from build123d import *

# Parameters (mm, degrees)
SKETCH1_R               = 6.35
BOSS_EXTRUDE1_DEPTH     = 25.4
CUT_EXTRUDE2_DEPTH      = 27.940768363
CUT_EXTRUDE2_DEPTH_BACK = 12.7
SKETCH3_R               = 4
SKETCH6_R               = 4.0005
CUT_EXTRUDE5_DEPTH      = 12.7
SKETCH4_R               = 1.1303
CUT_EXTRUDE3_DEPTH      = 6.35
SKETCH7_R               = 3.175
CUT_EXTRUDE6_DEPTH      = 12.7


with BuildPart() as part:
    # Sketch1 → Boss-Extrude1 (new body)
    with BuildSketch(Plane(origin=(0, 0, 0), x_dir=(1, 0, 0), z_dir=(0, 1, 0))):
        with Locations(Location((0, 0, 0), (0, 0, 270))):
            Circle(SKETCH1_R)
    extrude(amount=BOSS_EXTRUDE1_DEPTH)

    # Sketch3 → Cut-Extrude2 (cut, two sides: drawn at the far end of the back side and taken through both)
    with BuildSketch(Plane.XZ.offset(-CUT_EXTRUDE2_DEPTH_BACK)):
        with Locations(Location((0, 0, 0), (0, 0, 90))):
            Circle(SKETCH3_R)
    extrude(amount=CUT_EXTRUDE2_DEPTH + CUT_EXTRUDE2_DEPTH_BACK, mode=Mode.SUBTRACT)

    # Sketch6 → Cut-Extrude5 (cut)
    with BuildSketch(Plane(origin=(0, 0, 0), x_dir=(-1, 0, 0), z_dir=(0, -1, 0))):
        with Locations(Location((0, 0, 0), (0, 0, 90))):
            Circle(SKETCH6_R)
    extrude(amount=-CUT_EXTRUDE5_DEPTH, mode=Mode.SUBTRACT)

    # Sketch4 → Cut-Extrude3 (cut)
    with BuildSketch(Plane.XY.offset(6.35)):
        with Locations((0, 6.35)):
            Circle(SKETCH4_R)
        with Locations((0, 19.05)):
            Circle(SKETCH4_R)
    extrude(amount=-CUT_EXTRUDE3_DEPTH, mode=Mode.SUBTRACT)

    # Sketch7 → Cut-Extrude6 (cut)
    with BuildSketch(Plane(origin=(0, 25.4, 0), x_dir=(1, 0, 0), z_dir=(0, 1, 0))):
        with Locations(Location((0, 0, 0), (0, 0, 270))):
            Circle(SKETCH7_R)
    extrude(amount=-CUT_EXTRUDE6_DEPTH, mode=Mode.SUBTRACT)


solid = part.part
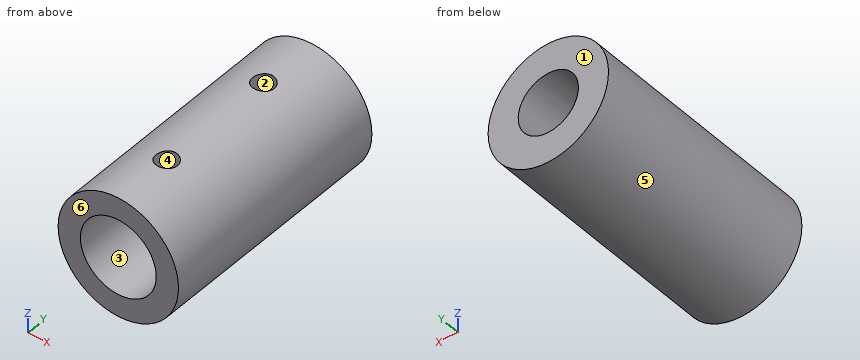
Work out the finished part from the listing and answer in its coordinate system (mm). Face numbers are marked on the shaded views. A direction names the side the tool comes from. Coordinates: 2 decimals unless noted, no trailing zeros. Write each loop counter-clockwise with the first axis right and the second up, starting at its lowest first coordinate (ties: lowest second). Pieces come first, ordered by that corner, then holes. Notation, with made-up numbers: M 24.5,-15 L 43.5,-15 A24 cw 43.5,17 Z; hole C 61.25,62 d4. An arc over 180 degrees is marked long. Answer as CSV lines item,"result". Start each with the question number.
Item 1: Section B-B on x = 0 is taken. Give the number of separate pieces and of enclosed holes in the cut face, and give its area (3 significant figures).
Item 2: Section C-C on y = 11.5 is taken. Write down the section's boundary in (x, z).
Item 3: Flat-ended cylindrical pins translate along their axes: P1, Ø4, axis at x = 0, z = 0, coming from the +Y side; P2, Ø3, axis at y = 13.5, z = -4.5, coming from the +X side; P3, Ø6.5, axis at x = -0.5, z = 2, coming from the -Y side; P4, Ø1.5, axis at y = 5, z = 4.5, coming from the +X side. Find the tip coordinate at first contact, or state that the pin passes through.
Item 4: Determine the mould class of the marked faces 4, 5 and 6 for opening direction X: released by +X, released by -X, zero draft, split by the parting line, or undercut.
Item 5: Consider L1, parallel to Y at x = 0, z = 5.1; L2, parallel to Y at x = 1, z = 5.75; L3, parallel to Y at x = 0, z = 3.75. Determine where each line is inside the solid, lowest interval first.
Item 6: A tool of negligible diameter and unlimited length cuts with its end or side. For the marked faces 1, 2 and 3, from which of +Z, -Z, +X, -X, +Y, -Y can it reach the whole face along a straight path? Write none if from no direction.
Item 7: Section D-D on x = -2.5 is taken. Write down the section's boundary in (y, z).
Checks:
1,separate pieces,"4"
1,enclosed holes,"0"
1,area,"128 mm²"
2,outline,"C 0,0 d12.7; hole C 0,0 d8"
3,P1,"passes through"
3,P2,"stops at x = 5.6"
3,P3,"stops at y = 0"
3,P4,"stops at x = 5.12"
4,face 4,"undercut"
4,face 5,"split by the parting line"
4,face 6,"zero draft"
5,L1,"y = 0 to 5.22, 7.48 to 17.92, 20.18 to 25.4"
5,L2,"y = 0 to 5.82, 6.88 to 18.52, 19.58 to 25.4"
5,L3,"y = 12.7 to 17.92, 20.18 to 25.4"
6,face 1,"+Z, -Z, +X, -X, +Y"
6,face 2,"+Z"
6,face 3,"-Y"
7,outline,"M 0,-5.84 L 25.4,-5.84 L 25.4,-1.96 L 12.7,-1.96 L 12.7,-3.12 L 0,-3.12 Z; M 0,3.12 L 12.7,3.12 L 12.7,1.96 L 25.4,1.96 L 25.4,5.84 L 0,5.84 Z"
